Here's how the part is built. I have some questions about the finished solid (model axes, mm). Round coordinates to 2 decimals unless told otherwise and drop trailing zeros. Loops run counter-clockwise (first coordinate to the right, second up) from the corner with the lowest first, then second, coordinate; pieces in that order, holes last. Notation, with made-up numbers: (84.25, -34) - (120.25, -34) arc R16 cw to (120.25, -23) - close; hole circle Ø5 at (-27.5, -38). An arc over 180 degrees is marked (long way). Answer as a JSON object with one key per item and string values. Group by question number.
1) If I drill on line 1 along X through (y, z) = (-25, 2.5); line 2 along Y through (x, z) = (-24.5, 7), over which ranges is the centre line in solid material (lowest first)? Write a range as [from, to].
2) Will these pins go through, and if not, where does the flat tip stop? P1, Ø1.8, axis at x = 0, y = 0, coming from the +Z side; P2, Ø4.5, axis at x = 25, y = 25, coming from the +Z side; P3, Ø5.5, axis at x = -25, y = 25, coming from the +Z side.
3) If we mould it in two halves opening along X, with no side actions, what happens to faces 1 (the face through (-1, 50, 4)), 2 (the face through (50, -1, 4)), 3 (the face through (-50, -1, 4)), 4 (the face through (-25.51, 23.38, 3.84))? For each: pulls with the +X half, pulls with the -X half, needs draft (parallel to the pull), parting line crosses it, or undercut.
4) I want a section at A-A, the plane x = -25. Please give me the cut outline in (y, z) (3 decimals).
from build123d import *

# Parameters (mm, degrees)
SKETCH_1_W                  = 100
SKETCH_1_H                  = 100
EXTRUDE_1_DEPTH             = 9
HOLE_WIZARD_M3_1_AT_2_COUNT = 2
HOLE_WIZARD_M3_1_AT_2_PITCH = 50
HOLE_WIZARD_M3_1_AT_3_COUNT = 2
HOLE_WIZARD_M3_1_AT_3_PITCH = 70.710678119
HOLE_WIZARD_M3_1_AT_4_COUNT = 2
HOLE_WIZARD_M3_1_AT_4_PITCH = 50


with BuildPart() as part:
    # 草圖1 → 填料-伸長1 (new body)
    with BuildSketch(Plane.XY):
        Rectangle(SKETCH_1_W, SKETCH_1_H)
    extrude(amount=EXTRUDE_1_DEPTH)

    # 草圖4 → M3 平頭機械螺釘的錐孔1 (revolve, cut)
    with BuildSketch(Plane(origin=(-25, 25, 9), x_dir=(0, -1, 0), z_dir=(1, 0, 0))):
        Polygon((0, 0), (0, 9), (1.725, 9), (1.7, 8.975), (1.7, 1.45), (3.15, 0), align=None)
    hole_wizard_m3_1 = revolve(axis=Axis((-25, 25, 15.35), (0, 0, -1)), mode=Mode.SUBTRACT)

    # M3 平頭機械螺釘的錐孔1 at 2: M3 平頭機械螺釘的錐孔1 ×2
    with Locations(*[(i * HOLE_WIZARD_M3_1_AT_2_PITCH, 0, 0) for i in range(1, HOLE_WIZARD_M3_1_AT_2_COUNT)]):
        add(hole_wizard_m3_1, mode=Mode.SUBTRACT)

    # M3 平頭機械螺釘的錐孔1 at 3: M3 平頭機械螺釘的錐孔1 ×2
    with Locations(*[Vector(0.7071067811865476, -0.7071067811865475, 0) * (i * HOLE_WIZARD_M3_1_AT_3_PITCH) for i in range(1, HOLE_WIZARD_M3_1_AT_3_COUNT)]):
        add(hole_wizard_m3_1, mode=Mode.SUBTRACT)

    # M3 平頭機械螺釘的錐孔1 at 4: M3 平頭機械螺釘的錐孔1 ×2
    with Locations(*[(0, -i * HOLE_WIZARD_M3_1_AT_4_PITCH, 0) for i in range(1, HOLE_WIZARD_M3_1_AT_4_COUNT)]):
        add(hole_wizard_m3_1, mode=Mode.SUBTRACT)

    # 草圖8 → Ø2.0mm 定位孔2 (revolve, cut)
    with BuildSketch(Plane(origin=(0, 0, 9), x_dir=(0, -1, 0), z_dir=(1, 0, 0))):
        Polygon((0, 0), (0, 6), (1, 5.399139381), (1, 0), align=None)
    revolve(axis=Axis((0, 0, 15.35), (0, 0, -1)), mode=Mode.SUBTRACT)


solid = part.part
Outcome:
{
 "1": {"line 1": "[-50, -26.7], [-23.3, 23.3], [26.7, 50]", "line 2": "[-50, -26.62], [-23.38, 23.38], [26.62, 50]"},
 "2": {"P1": "z = 3.54", "P2": "z = 8.1", "P3": "z = 8.6"},
 "3": {"face 1": "needs draft", "face 2": "pulls with the +X half", "face 3": "pulls with the -X half", "face 4": "undercut"},
 "4": {"outline": "(-50, 0) - (-26.725, 0) - (-26.7, 0.025) - (-26.7, 7.55) - (-28.15, 9) - (-50, 9) - close; (-23.3, 0.025) - (-23.275, 0) - (23.275, 0) - (23.3, 0.025) - (23.3, 7.55) - (21.85, 9) - (-21.85, 9) - (-23.3, 7.55) - close; (26.7, 0.025) - (26.725, 0) - (50, 0) - (50, 9) - (28.15, 9) - (26.7, 7.55) - close"}
}
